```python
from build123d import *

# Parameters (mm, degrees)
SKETCH_W    = 80
SKETCH_H    = 88
SKETCH_R    = 3
PAD_DEPTH   = 10
FILLET_R    = 10
FILLET001_R = 1


with BuildPart() as part:
    # Sketch → Pad (new body)
    with BuildSketch(Plane.XY):
        with Locations((15, -15)):
            Rectangle(SKETCH_W, SKETCH_H)
        with Locations((-10, -52)):
            Circle(SKETCH_R, mode=Mode.SUBTRACT)
        with Locations((40, -52)):
            Circle(SKETCH_R, mode=Mode.SUBTRACT)
        with Locations((40, 22)):
            Circle(SKETCH_R, mode=Mode.SUBTRACT)
        with Locations((-10, 22)):
            Circle(SKETCH_R, mode=Mode.SUBTRACT)
        with BuildLine():
            ThreePointArc((-5, -6.244998), (8, 0), (-5, 6.244998))
            Line((-5, 6.244998), (-5, 10))
            ThreePointArc((-5, 10), (-7, 12), (-9, 10))
            Line((-9, 10), (-9, -10))
            ThreePointArc((-9, -10), (-7, -12), (-5, -10))
            Line((-5, -6.244998), (-5, -10))
        make_face(mode=Mode.SUBTRACT)
    extrude(amount=PAD_DEPTH)

    # Fillet
    fillet_edges = [part.edges().sort_by_distance(p)[0] for p in [
        (-25, -59, 5),
        (-25, 29, 5),
    ]]
    fillet(fillet_edges, radius=FILLET_R)

    # Fillet001
    fillet001_edges = [part.edges().sort_by_distance(p)[0] for p in [
        (55, -59, 5),
        (55, 29, 5),
    ]]
    fillet(fillet001_edges, radius=FILLET001_R)


solid = part.part
```
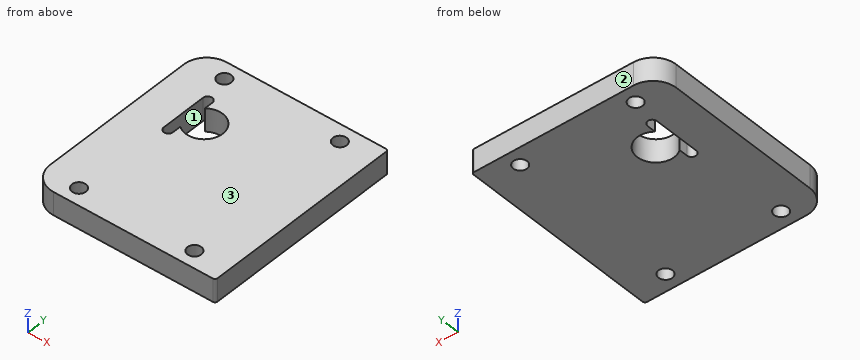
Source: CAD feature listing. Evaluate the final solid. Frame: model axes, mm. Face numbers are marked on the shaded views. Coordinates: 2 decimals unless noted, no trailing zeros. Loops run counter-clockwise (first coordinate to the right, second up) from the corner with the lowest first, then second, coordinate; pieces in that order, holes last. Notation, with made-up numbers: M 23.25,-24.5 L 78.25,-24.5 A18 ccw 78.25,-6.5 Z; hole C 18.5,24 d7. An arc over 180 degrees is marked long. Use a Markdown table: item, result. Add a question column.
Q1. Section query D-D, the plane x = 3.5. Return loops of the section in (y, z), and give its area (3 significant figures).
Q2. Section query B-B, the plane z = 1.25. Return loops of the section in (x, y) (3 decimals).
Q3. Material intervals for L1, parallel to Y at x = -10, z = 7.5; L2, parallel to Y at x = 0, z = 3.5; L3, parallel to X at y = 21.5, z = 3.5, sorted ascending.
Q4. Draft query along Y for the marked faces 1, 2 and 3. Return one class per face: pulls with the +Y half, pulls with the -Y half, needs draft (parallel to the pull), parting line crosses it, or undercut.
Q5. Section query C-C, the plane y = 22. Return loops of the section in (x, z), and give its area (3 significant figures).
Q6. Section query A-A, the plane x = 40. Return loops of the section in (y, z).
Result:
| question | item | result |
|---|---|---|
| 1 | outline | M -59,0 L -7.19,0 L -7.19,10 L -59,10 Z; M 7.19,0 L 29,0 L 29,10 L 7.19,10 Z |
| 1 | area | 736 mm2 |
| 2 | outline | M -25,-49 A10 ccw -15,-59 L 54,-59 A1 ccw 55,-58 L 55,28 A1 ccw 54,29 L -15,29 A10 ccw -25,19 Z; hole C -10,-52 d6; hole C -10,22 d6; hole M -9,-10 A2 ccw -5,-10 L -5,-6.245 A8 ccw long -5,6.245 L -5,10 A2 ccw -9,10 Z; hole C 40,-52 d6; hole C 40,22 d6 |
| 3 | L1 | y = -59 to -55, -49 to 19, 25 to 29 |
| 3 | L2 | y = -59 to -8, 8 to 29 |
| 3 | L3 | x = -24.68 to -12.96, -7.04 to 37.04, 42.96 to 55 |
| 4 | face 1 | undercut |
| 4 | face 2 | pulls with the +Y half |
| 4 | face 3 | needs draft |
| 5 | outline | M -24.54,0 L -13,0 L -13,10 L -24.54,10 Z; M -7,0 L 37,0 L 37,10 L -7,10 Z; M 43,0 L 55,0 L 55,10 L 43,10 Z |
| 5 | area | 675 mm2 |
| 6 | outline | M -59,0 L -55,0 L -55,10 L -59,10 Z; M -49,0 L 19,0 L 19,10 L -49,10 Z; M 25,0 L 29,0 L 29,10 L 25,10 Z |
